Drawing for the job (mm, zero at the part's lowest x, y, z). A direction names the side the tool comes from. Round coordinates to 2 decimals unless told otherwise and drop trailing zeros. Write each loop counter-clockwise with the first axis right and the second up, starting at its lowest first coordinate (ties: lowest second). Pieces come first, ordered by that corner, then holes. Notation, with made-up numbers: M -18.5,-32 L 20.5,-32 A14 cw 20.5,-11 Z; hole C 88.25,61.5 d5. An arc over 180 degrees is marked long. Use a Markdown table: item, result.
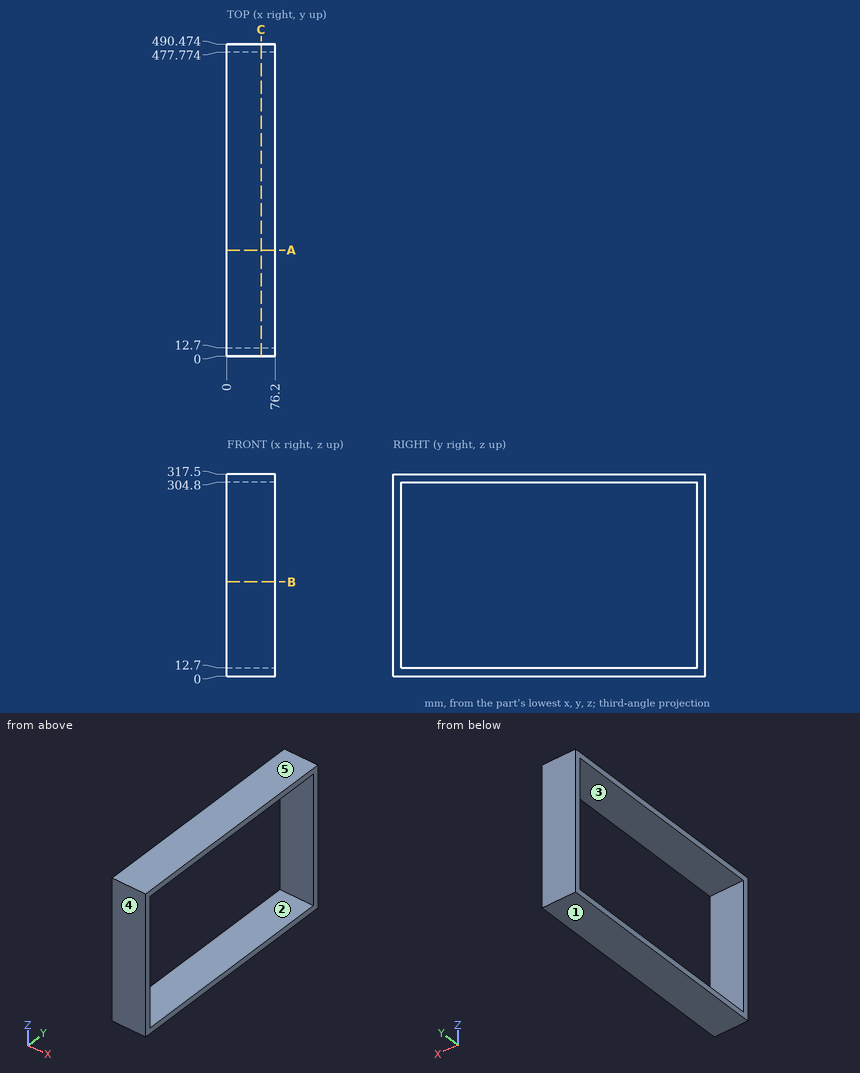
Q1. Cut at A-A on y = 166.5. Give the cut face in (x, z), and give its area (3 significant figures).
Response values:
| item | result |
|---|---|
| outline | M 0,0 L 76.2,0 L 76.2,12.7 L 0,12.7 Z; M 0,304.8 L 76.2,304.8 L 76.2,317.5 L 0,317.5 Z |
| area | 1,940 mm2 |
Q2. Cut at C-C on x = 54. Give the cut face in (y, z), and give its area (3 significant figures).
Response values:
| item | result |
|---|---|
| outline | M 0,0 L 490.47,0 L 490.47,317.5 L 0,317.5 Z; hole M 12.7,12.7 L 477.77,12.7 L 477.77,304.8 L 12.7,304.8 Z |
| area | 19,900 mm2 |
Q3. Cut at B-B on z = 148. Give the cut face in (x, y), and give its area (3 significant figures).
Response values:
| item | result |
|---|---|
| outline | M 0,0 L 76.2,0 L 76.2,12.7 L 0,12.7 Z; M 0,477.77 L 76.2,477.77 L 76.2,490.47 L 0,490.47 Z |
| area | 1,940 mm2 |
Q4. Two-plate mould, pull along Y, no slides. Class the marked faces 3, 4 and 5: +Y half, -Y half, draft (parallel to the pull), parting line (faces both ways), or undercut.
Response values:
| item | result |
|---|---|
| face 3 | undercut |
| face 4 | -Y half |
| face 5 | draft |
Q5. Which spindle directions (+Z, -Z, +X, -X, +Y, -Y) get a long thin tool onto all of the face, cutting with end or side? Do the marked faces 1 and 2. Say none if no direction does.
Response values:
| item | result |
|---|---|
| face 1 | -Z, +X, -X, +Y, -Y |
| face 2 | +X, -X |
Q6. Drill centre lines: L1, parallel to Y at x = 46, z = 227; L2, parallel to Z at x = 44, y = 359.5. Where is each one in solid material? Low to high.
Response values:
| item | result |
|---|---|
| L1 | y = 0 to 12.7, 477.77 to 490.47 |
| L2 | z = 0 to 12.7, 304.8 to 317.5 |
